```python
from build123d import *

# Parameters (mm, degrees)
SKETCH1_R           = 76.1746
SKETCH1_R_2         = 3.175
BOSS_EXTRUDE1_DEPTH = 9.525
CIRPATTERN1_COUNT   = 4


with BuildPart() as part:
    # Sketch1 → Boss-Extrude1 (new body)
    with BuildSketch(Plane(origin=(0, 0, 0), x_dir=(1, 0, 0), z_dir=(0, 1, 0))):
        with Locations(Location((0, 0, 0), (0, 0, 90))):
            Circle(SKETCH1_R)
        with Locations(Location((0, 0, 0), (0, 0, 90))):
            Circle(SKETCH1_R_2, mode=Mode.SUBTRACT)
    extrude(amount=BOSS_EXTRUDE1_DEPTH)

    # Sketch3 → Tap Drill for #6-32 Tap1 (revolve, cut)
    with BuildSketch(Plane(origin=(0, 4.7625, -76.1746), x_dir=(0, 1, 0), z_dir=(1, 0, 0))):
        Polygon((0, 0), (0, 10.46469403), (1.35255, 9.652), (1.35255, 0), align=None)
    tap_drill_for_6_32_tap1 = revolve(axis=Axis((0, 4.7625, -82.5246), (0, 0, 1)), mode=Mode.SUBTRACT)

    # CirPattern1: Tap Drill for #6-32 Tap1 ×4 about axis
    cirpattern1_axis = Axis((0, 9.525, 0), (0, 1, 0))
    for i in range(1, CIRPATTERN1_COUNT):
        add(tap_drill_for_6_32_tap1.rotate(cirpattern1_axis, i * 360 / CIRPATTERN1_COUNT), mode=Mode.SUBTRACT)


solid = part.part
```
Work out the finished part from the listing and answer in its coordinate system (mm). Give positions to 0.01 mm unless a question says otherwise; leave off trailing zeros. Loops run counter-clockwise (first coordinate to the right, second up) from the corner with the lowest first, then second, coordinate; pieces in that order, holes last. Notation, with made-up numbers: (64.25, 38.5) -> (102.25, 38.5) arc R27 cw to (102.25, 71.5) -> close; hole circle Ø2 at (33.25, 23). An arc over 180 degrees is marked (long way). Put each result on its own line as item: value. Start each with the question number.
Item 1: The part is cut by section B-B (x = -30). Give the vertices of the cut face in (y, z) (3 decimals).
Item 2: The mould has two halves that part along X. Classify faces 1 (the face through (16, 9.525, 1)), 2 (the face through (1.93, 4.7, 2.52)), 3 (the face through (-22.881, 4.696, -72.657)): released by +X, released by -X, zero draft, split by the parting line, or undercut.
Item 3: Find the intervals of material crossed by L1, parallel to X at y = 2.5, z = 0 (3 decimals); L2, parallel to Y at x = -70, z = 0 (3 decimals); L3, parallel to Z at x = -1, y = 0.5, in increasing order. Write a range as [from, to].
Item 4: The part is cut by section A-A (z = 22). Give the vertices of the cut face in (x, y) (3 decimals), then the cut area to 3 significant figures.
Item 5: Each of these flat-tipped pins is pushed along its axis until it touches: P1, Ø1.6, axis at y = 4.76, z = 0, coming from the -X side; P2, Ø5, axis at x = 42, y = 6, coming from the -Z side; P3, Ø2.5, axis at y = 4.76, z = 0, coming from the -X side; P4, Ø5, axis at x = 0, z = 0, coming from the -Y side. Where does it stop, or does it pass through?
Answers below:
1. outline: (0, -70.018) -> (9.525, -70.018) -> (9.525, 70.018) -> (0, 70.018) -> close
2. face 1: zero draft
2. face 2: undercut
2. face 3: split by the parting line
3. L1: [-76.175, -3.175], [3.175, 76.175]
3. L2: [0, 3.41], [6.115, 9.525]
3. L3: [-76.17, -3.01], [3.01, 76.17]
4. outline: (-72.929, 0) -> (72.929, 0) -> (72.929, 9.525) -> (-72.929, 9.525) -> close
4. area: 1,390 mm2
5. P1: x = -66.19
5. P2: z = -65.13
5. P3: x = -66.46
5. P4: through
